Autodesk Inventor part; units mm, degrees
ref_plane "Начальная плоскость" through (0, 0, 16.5685) normal (0, 0, 1) x (1, 0, 0)
ref_plane "Конечная плоскость" through (0, 0, 486.57) normal (0, 0, 1) x (1, 0, 0)
ref_plane "РабПлоскость4" through (43.57, -128.2843, -71.7157) normal (0, 0.7071, -0.7071) x (1, 0, 0)
ref_plane "Начальная плоскость" through (0, 0, 16.5685) normal (0, 0, 1) x (1, 0, 0)
ref_plane "Конечная плоскость" through (0, 0, 486.57) normal (0, 0, 1) x (1, 0, 0)
sketch "Эскиз" plane through (0, 0, 0) normal (0, 0, 1) x (1, 0, 0)
  line L0 (-1.43, 0) -> (-1.43, 40)
  line L1 (-1.43, 40) -> (43.57, 40)
  line L2 (43.57, 40) -> (43.57, 38.1774)
  line L3 (39.9881, 34.1993) -> (11.2338, 31.1771)
  line L4 (4.07, 23.221) -> (4.07, 0)
  line L5 (4.07, 0) -> (-1.43, 0) construction
  line L6 (23.82, 40) -> (23.82, 32.5) construction
  line L7 (43.57, 34.5758) -> (43.57, 32.5) construction
  line L8 (43.57, 32.5) -> (23.82, 32.5) construction
  line L9 (0, 15) -> (0, -27) construction
  line L10 (-5.539, 0) -> (16.0067, 0) construction
  line L11 (-1.43, 0) -> (-1.43, -40)
  line L12 (-1.43, -40) -> (43.57, -40)
  line L13 (43.57, -40) -> (43.57, -38.1774)
  line L14 (39.9881, -34.1993) -> (11.2338, -31.1771)
  line L15 (4.07, -23.221) -> (4.07, 0)
  arc A0 (11.2338, 31.1771) -> (4.07, 23.221) centre (12.07, 23.221) ccw
  arc A1 (4.07, -23.221) -> (11.2338, -31.1771) centre (12.07, -23.221) ccw
  arc A2 (39.9881, 34.1993) -> (43.57, 38.1774) centre (39.57, 38.1774) ccw
  arc A3 (43.57, -38.1774) -> (39.9881, -34.1993) centre (39.57, -38.1774) ccw
  line L16 (0, 56) -> (0, -56) construction
  line L17 (-15.5135, 0) -> (54.308, 0) construction
  point P0 (4.07, 30.4242)
  point P1 (43.57, -34.5758)
  point P2 (4.07, -30.4242)
  point P3 (23.82, -40)
  point P4 (23.82, -32.5)
  dimension "d0" = 5.5
  dimension "d1" = 40
  dimension "d2" = 45
  dimension "d3" = 7.5
  dimension "d4" = 19.75
  dimension "d5" = 2.0758
  dimension "d23" = 8
  dimension "d24" = 4
  dimension "d25" = 1.43
extrude "Тело" add sketch "Эскиз" along normal up to surface (470.0015 mm away) from surface at 16.5685
sketch "Sketch3" plane through (0, 0, 0) normal (0, 0, 1) x (1, 0, 0)
  line L0 (0, 0) -> (10, 0)
ref_plane "Work Plane3" through (0, 0, 0) normal (0, -1, 0) x (1, 0, 0)
sketch "Sketch4" plane through (0, 0, 0) normal (0, -1, 0) x (1, 0, 0)
  line L0 (-2, 16.5685) -> (12, 16.5685)
  line L1 (-2, 486.57) -> (12, 486.57)
  dimension "d29" = 470.0015
ref_plane "РабПлоскость4" through (43.57, -128.2843, -71.7157) normal (0, 0.7071, -0.7071) x (1, 0, 0)
split "Разделение1" plane through (43.57, -128.2843, -71.7157) removes the side toward (0, 0.7071, -0.7071)
ref_plane "РабПлоскость5" through (43.57, 220, 486.57) normal (0, 0, 1) x (1, 0, 0)
split "Разделение2" plane through (43.57, 220, 486.57) removes the side toward (0, 0, 1)
equation "\"d0\" = G_T"
equation "\"d1\" = 0.5 * G_H"
equation "\"d2\" = G_W"
equation "\"d3\" = G_T1"
equation "\"d4\" = G_C"
equation "\"d23\" = G_IR"
equation "\"d24\" = G_ER"
equation "\"d25\" = ex"
equation "\"d6\" = G_L"
equation "\"G_W\" = 45"
equation "\"G_T\" = 5.5"
equation "\"G_T1\" = 7.5"
equation "\"G_NG\" = 0.105104"
equation "\"G_ER\" = 4"
equation "\"G_IR\" = 8"
equation "\"G_C\" = 19.75"
equation "\"G_L\" = d29"
equation "\"ex\" = 1.43"
equation "\"G_OFFSET_START\" = -16.56854"
equation "\"d26\" = -G_OFFSET_START"
equation "\"d27\" = G_OFFSET_END + B_L"
equation "\"B_L\" = 526.57"
properties part number "ISO 657/11 - CH 80 x 8 - 470" material "Сталь, мягкая"
The listing builds one solid part. Answer for the finished solid, in the listing's coordinates (mm). A direction names the side the tool comes from. Give positions to 0.01 mm unless a question says otherwise; leave off trailing zeros. Order: outer loops, then holes, each group sorted by start corner. A loop starts at its lowest first (then second) coordinate and runs counter-clockwise, first axis right, second up. Notation, with made-up numbers: (25, 59) - (41, 59) arc R24 cw to (41, 97) - close; hole circle Ø9 at (48, 10). An arc over 180 degrees is marked (long way). Answer in a Markdown table with one row per item. Add a question column.
Q1. The part is cut by section D-D (z = 73). Determine the outline of the cut face in (x, y).
Q2. The part is cut by section C-C (y = -16). Determine the outline of the cut face in (x, z), then the cut area to 3 significant figures.
Q3. Which of the six approach directions +Z, -Z, +X, -X, +Y, -Y give full straight-line access (tool end or side, diameter ignored) to faces 1 (the cylindrical face through (6.07, 28.51, 280.33)), 2 (the flat face through (21, -40, 248))?
Q4. The part is cut by section A-A (x = 28.5). Determine the outline of the cut face in (y, z), then the cut area to 3 significant figures.
Q5. The part is cut by section B-B (z = 364). Determine the outline of the cut face in (x, y).
Q6. For a pull along Y with two mould halves and no side action, classify faces 3 (the flat face through (-1.43, -1, 248)), 4 (the flat face through (2.63, 0.19, 56.76)), 5 (the cylindrical face through (6.18, -28.635, 252.753)) as released by +Y, released by -Y, zero draft, split by the parting line, or undercut.
Q7. Given P1, Ø14, axis at y = 11, z = 155.5, coming from the +X side; P2, Ø6, axis at x = 24, z = 78.5, coming from the +Y side, each flat-ended and moving along its own axis, determine where each tip first touches the part or whether it passes through.
Q8. Find the intervals of material crossed by line 1 along X through (y, z) = (9, 79); line 2 along Y through (x, z) = (39.5, 60.5); line 3 along Y through (x, z) = (6, 250.5), in increasing order. Write a range as [from, to].
Determined:
| question | item | result |
|---|---|---|
| 1 | outline | (-1.43, -40) - (43.57, -40) - (43.57, -38.18) arc R4 ccw to (39.99, -34.2) - (11.23, -31.18) arc R8 cw to (4.07, -23.22) - (4.07, 16.43) - (-1.43, 16.43) - close |
| 2 | outline | (-1.43, 40.57) - (4.07, 40.57) - (4.07, 486.57) - (-1.43, 486.57) - close |
| 2 | area | 2,450 mm² |
| 3 | face 1 | +Z, -Z, +X |
| 3 | face 2 | +Z, -Z, +X, -X, -Y |
| 4 | outline | (-40, 16.57) - (-32.99, 23.58) - (-32.99, 486.57) - (-40, 486.57) - close; (32.99, 89.56) - (40, 96.57) - (40, 486.57) - (32.99, 486.57) - close |
| 4 | area | 6,030 mm² |
| 5 | outline | (-1.43, -40) - (43.57, -40) - (43.57, -38.18) arc R4 ccw to (39.99, -34.2) - (11.23, -31.18) arc R8 cw to (4.07, -23.22) - (4.07, 23.22) arc R8 cw to (11.23, 31.18) - (39.99, 34.2) arc R4 ccw to (43.57, 38.18) - (43.57, 40) - (-1.43, 40) - close |
| 6 | face 3 | zero draft |
| 6 | face 4 | released by +Y |
| 6 | face 5 | undercut |
| 7 | P1 | stops at x = 4.07 |
| 7 | P2 | stops at y = -32.2 |
| 8 | line 1 | x = [-1.43, 4.07] |
| 8 | line 2 | y = [-40, -34.15] |
| 8 | line 3 | y = [-40, -28.43], [28.43, 40] |
